Check sheet for the modelled part. Datum: model origin and axes. Units: mm. Face numbers are marked on the shaded views. Round coordinates to 2 decimals unless told otherwise and drop trailing zeros. Write each loop counter-clockwise with the first axis right and the second up, starting at its lowest first coordinate (ties: lowest second). Pieces come first, ordered by that corner, then holes.
from build123d import *

# Parameters (mm, degrees)
F1_DEPTH = 12.7
F3_D     = 254


with BuildPart() as f1:
    # F0 (on Top) → F1 (new body)
    with BuildSketch(Plane.XY):
        Polygon((344.057809, 313.70795), (13.857809, 313.70795), (13.857809, 262.90795), (-36.942191, 262.90795), (-36.942191, 34.30795), (13.857809, 34.30795), (13.857809, -16.49205), (344.057809, -16.49205), (344.057809, 34.30795), (394.857809, 34.30795), (394.857809, 262.90795), (344.057809, 262.90795), align=None)
    extrude(amount=F1_DEPTH)

    # F3 (through all)
    with Locations(Plane.XY.offset(12.7)):
        with Locations((178.957809, 148.60795)):
            Hole(F3_D / 2)


solid = f1.part
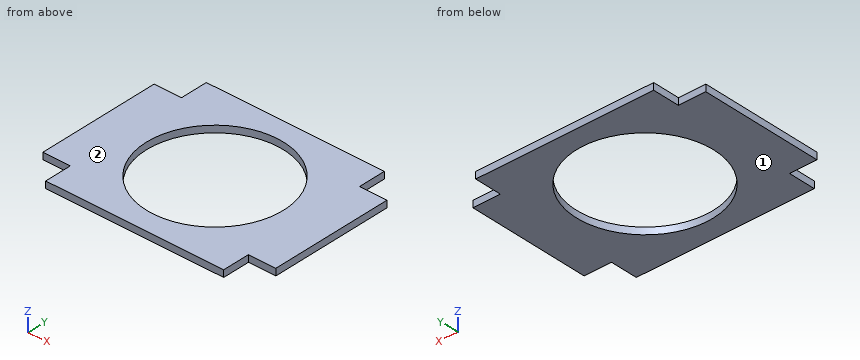
1. Scan lines: line 1 along X through (y, z) = (13, 3.25); line 2 along Y through (x, z) = (-1, 5.5); line 3 along Y through (x, z) = (61.5, 8.5). Record each from-to range of solid material in increasing order.
2. Sectioned sample at A-A, the plane x = 287.5. Enter the section's corners in (y, z).
3. Go/stop test with flat-tipped pins: pin 1 (4 mm diameter, centred on x = -20, z = 3.5, fed in from -Y); pin 2 (4 mm diameter, centred on y = 293, z = 4, fed in from +X). Record where each tip stops, or that it passes through.
4. Sectioned sample at D-D, the plane y = 9.5. Enter the section's corners in (x, z).
5. Release check for a two-part mould opening along Z. For the marked faces 1 and 2 record: released by +Z, released by -Z, zero draft, split by the parting line, or undercut.
6. Sectioned sample at B-B, the plane y = 75. Enter the section's corners in (x, z), plus the area to 3 significant figures.
7. Sectioned sample at C-C, the plane z = 2.5. Enter the section's corners in (x, y), plus the area to 3 significant figures.
Computed values:
1. line 1: x = 13.86 to 344.06
1. line 2: y = 34.31 to 262.91
1. line 3: y = -16.49 to 100.31, 196.91 to 313.71
2. outline: (-16.49, 0) - (82.67, 0) - (82.67, 12.7) - (-16.49, 12.7) - close; (214.54, 0) - (313.71, 0) - (313.71, 12.7) - (214.54, 12.7) - close
3. pin 1: stops at y = 34.31
3. pin 2: stops at x = 344.06
4. outline: (13.86, 0) - (344.06, 0) - (344.06, 12.7) - (13.86, 12.7) - close
5. face 1: released by -Z
5. face 2: released by +Z
6. outline: (-36.94, 0) - (75.46, 0) - (75.46, 12.7) - (-36.94, 12.7) - close; (282.45, 0) - (394.86, 0) - (394.86, 12.7) - (282.45, 12.7) - close
6. area: 2,860 mm2
7. outline: (-36.94, 34.31) - (13.86, 34.31) - (13.86, -16.49) - (344.06, -16.49) - (344.06, 34.31) - (394.86, 34.31) - (394.86, 262.91) - (344.06, 262.91) - (344.06, 313.71) - (13.86, 313.71) - (13.86, 262.91) - (-36.94, 262.91) - close; hole circle Ø254 at (178.96, 148.61)
7. area: 81,600 mm2
